Here's how the part is built. I have some questions about the finished solid (model axes, mm). A direction names the side the tool comes from. Coordinates: 2 decimals unless noted, no trailing zeros. Write each loop counter-clockwise with the first axis right and the second up, starting at its lowest first coordinate (ties: lowest second). Pieces come first, ordered by that corner, then holes. Notation, with made-up numbers: (80, 36.5) - (94, 36.5) arc R33 cw to (94, 74.5) - close; hole circle Ø6 at (18, -27). An arc over 180 degrees is marked (long way). Answer in a Markdown table with one row per item. Add a question column.
Item 1: If I drill on probe 1 along Z at (x, y) = (13, 0); probe 2 along Z at (x, y) = (16.5, -24); probe 3 along X at (y, z) = (-33, -0.2), over which ranges is the centre line in solid material (lowest first)? Write a range as from..to.
Item 2: Imagine slicing it at C-C (x = 18.5). Please give me the cut outline in (y, z), plus the area to 3 significant figures.
Item 3: Imagine slicing it at B-B (y = 0). Please give me the cut outline in (x, z).
Item 4: Which directions (+Z, -Z, +X, -X, +Y, -Y) give clear straight access to the entire face, cutting with the end or side of a thin tool? Please do faces 1 (the face through (15.003, -46.442, 0.007)), 2 (the face through (1, 0.649, 0.624)), 3 (the face through (23, 0.649, -0.624)).
Item 5: We'd pull the mould along X, two halves only. Please class faces 4 (the face through (24.83, -30.27, 0.01)), 5 (the face through (12, -31, 0.5)), 6 (the face through (9.08, -46.06, 0.01)): +X half, -X half, draft (parallel to the pull), parting line (faces both ways), or undercut.
Item 6: I'm going to push flat-ended pins straight in: pin 1 (1.5 mm diameter, centred on x = 7, y = -4.5, fed in from +Z); pin 2 (5 mm diameter, centred on x = 13.5, y = -36, fed in from -Z); pin 3 (1.4 mm diameter, centred on y = -0.5, z = -0.5, fed in from -X). Where does each tip first touch, or does it pass through?
Item 7: Imagine slicing it at A-A (z = 0). Please give me the cut outline in (x, y).
Item 8: Imagine slicing it at D-D (y = -44). Please give me the cut outline in (x, z), plus the area to 3 significant figures.
from build123d import *

# Parameters (mm, degrees)
F0_R      = 1.45
F1_DEPTH  = 24
F5_DEPTH  = 65
F7_DEPTH  = 25
F8_W      = 31
F8_H      = 5
F9_DEPTH  = 25
F10_R     = 0.75
F11_DEPTH = 40
F12_W     = 1
F12_H     = 2.9
F12_H_2   = 3.020188
F13_DEPTH = 12.5


with BuildPart() as f1:
    # F0 (on Right) → F1 (new body)
    with BuildSketch(Plane.YZ):
        Circle(F0_R)
    extrude(amount=F1_DEPTH)

    # F4 (on offset) → F5 (join)
    with BuildSketch(Plane.XZ.offset(65)):
        Polygon((22.5, 0.5), (1.5, 0.5), (-3.5, 0.5), (-3.5, -0.5), (1.5, -0.5), (22.5, -0.5), (27.5, -0.5), (27.5, 0.5), align=None)
    extrude(amount=-F5_DEPTH)

    # F6 (on face) → F7 (cut)
    with BuildSketch(Plane.XY.offset(0.5)):
        Polygon((27.5, -65), (27.5, 0), (24, 0), (24, -1.361066), (22.604697, -1.361066), align=None)
        Polygon((0, 0), (-3.5, 0), (-3.5, -65), (1.395303, -1.361066), (0, -1.361066), align=None)
        Polygon((5, -65), (12, -65), (19, -65), (12, -32.5), align=None)
    extrude(amount=-F7_DEPTH, mode=Mode.SUBTRACT)

    # F8 (on face) → F9 (cut)
    with BuildSketch(Plane.XY.offset(0.5)):
        with Locations((12, -62.5)):
            Rectangle(F8_W, F8_H)
    extrude(amount=-F9_DEPTH, mode=Mode.SUBTRACT)

    # F10 (on face) → F11 (cut)
    with BuildSketch(Plane.YZ.offset(24)):
        Circle(F10_R)
    extrude(amount=-F11_DEPTH, mode=Mode.SUBTRACT)

    # F12 (on Top) → F13 (cut, symmetric)
    with BuildSketch(Plane.XY):
        with Locations((0.5, 0)):
            Rectangle(F12_W, F12_H)
        with Locations((23.5, -0.060094)):
            Rectangle(F12_W, F12_H_2)
    extrude(amount=F13_DEPTH, both=True, mode=Mode.SUBTRACT)


solid = f1.part
Here are the results:
| question | item | result |
|---|---|---|
| 1 | probe 1 | z = -1.45..-0.75, 0.75..1.45 |
| 1 | probe 2 | z = -0.5..0.5 |
| 1 | probe 3 | x = -1.04..11.89, 12.11..25.04 |
| 2 | outline | (-60, -0.5) - (-1.36, -0.5) arc R1.45 ccw (long way) to (-1.36, 0.5) - (-60, 0.5) - close; hole circle Ø1.5 at (0, 0) |
| 2 | area | 63.4 mm2 |
| 3 | outline | (1, -1.45) - (23, -1.45) - (23, -0.75) - (1, -0.75) - close; (1, 0.75) - (23, 0.75) - (23, 1.45) - (1, 1.45) - close |
| 4 | face 1 | +Z, -Z, -Y |
| 4 | face 2 | +Z, -Z, -X, +Y |
| 4 | face 3 | +Z, -Z, +X, +Y |
| 5 | face 4 | +X half |
| 5 | face 5 | draft |
| 5 | face 6 | undercut |
| 6 | pin 1 | stops at z = 0.5 |
| 6 | pin 2 | stops at z = -0.5 |
| 6 | pin 3 | stops at x = 1 |
| 7 | outline | (-3.12, -60) - (6.08, -60) - (12, -32.5) - (17.92, -60) - (27.12, -60) - (22.6, -1.36) - (23, -1.36) - (23, -0.75) - (1, -0.75) - (1, -1.36) - (1.4, -1.36) - close; (1, 0.75) - (23, 0.75) - (23, 1.45) - (1, 1.45) - close |
| 8 | outline | (-1.88, -0.5) - (9.52, -0.5) - (9.52, 0.5) - (-1.88, 0.5) - close; (14.48, -0.5) - (25.88, -0.5) - (25.88, 0.5) - (14.48, 0.5) - close |
| 8 | area | 22.8 mm2 |
